Autodesk Inventor part; units mm, degrees
ref_plane "Work Plane4" through (0, 0, -5) normal (0, 0, 1) x (1, 0, 0)
ref_plane "YZ Plane" through (0, 0, 0) normal (1, 0, 0) x (0, 1, 0)
ref_plane "XZ Plane" through (0, 0, 0) normal (0, 1, 0) x (-1, 0, 0)
sketch "Sketch1" plane through (0, 0, 0) normal (0, 0, 1) x (1, 0, 0)
  circle A0 centre (0, 0) radius 71.5
  circle A1 centre (0, 0) radius 73.5
  circle A2 centre (0, 0) radius 81.5
  circle A3 centre (0, 0) radius 83.5
  circle A4 centre (0, 0) radius 91.5
  circle A5 centre (0, 0) radius 93.5
  circle A6 centre (0, 0) radius 52.5
  circle A7 centre (0, 0) radius 62.5
  dimension "d0" = 143
  dimension "d1" = 147
  dimension "d2" = 163
  dimension "d3" = 167
  dimension "d4" = 183
  dimension "d5" = 187
  dimension "d6" = 105
  dimension "d7" = 125
extrude "Extrusion1" add sketch "Sketch1" along normal blind 10
extrude "Extrusion2" add sketch "Sketch1" against normal blind 10 contours A0 | A1 | A2 | A3 | A4 | A5 | A6 | A7
extrude "Extrusion3" cut sketch "Sketch1" against normal blind 10 contours A6
ref_plane "Work Plane4" through (0, 0, -5) normal (0, 0, 1) x (1, 0, 0)
ref_plane "Work Plane3" through (0, 0, 0) normal (0, 0, 1) x (1, 0, 0)
sketch "Sketch3" plane through (0, 0, 10) normal (0, 0, 1) x (1, 0, 0)
  circle A0 centre (0, 0) radius 61
  dimension "d18" = 122
sketch "Sketch4" plane through (0, 0, 5) normal (0, 0, 1) x (1, 0, 0)
  circle A0 centre (0, 0) radius 61
  dimension "d19" = 122
sketch "Sketch5" plane through (0, 0, 0) normal (0, 0, 1) x (1, 0, 0)
  circle A0 centre (0, 0) radius 61
  dimension "d20" = 122
ref_plane "Work Plane1" through (0, 0, 10) normal (0, 0, 1) x (1, 0, 0)
ref_plane "Work Plane2" through (0, 0, 5) normal (0, 0, 1) x (1, 0, 0)
properties part number "labyrinth"
Geometry: final body of the model. Coordinates: model frame, mm. A direction names the side the tool comes from. Coordinates: 2 decimals unless noted, no trailing zeros. Loops run counter-clockwise (first coordinate to the right, second up) from the corner with the lowest first, then second, coordinate; pieces in that order, holes last. Notation, with made-up numbers: (47, 60.25) -> (83, 60.25) arc R19 cw to (83, 72.25) -> close; hole circle Ø9 at (52.25, 0.25). An arc over 180 degrees is marked (long way). Use a Markdown table: item, result. Add a question column.
(1) Line query: line 1 along Y through (x, z) = (1.5, -2); line 2 along X through (y, z) = (-2, -5.5); line 3 along Z through (x, y) = (-9, -68.5). Output: solid intervals per line, ascending.
(2) Pin query (flat end, axial travel): pin 1 Ø3 at (y, z) = (58, 1.5) entering from +X; pin 2 Ø10 at (x, y) = (44.5, -22.5) entering from +Z; pin 3 Ø1 at (x, z) = (42.5, 1.5) entering from +Y; pin 4 Ø3 at (x, z) = (2.5, -3.5) entering from -Y. Return the tip coordinate at first contact, or that it passes through.
(3) Section query D-D, the plane y = -60. Return loops of the section in (x, z), plus the area to 3 significant figures.
(4) Access query for faces 4 (the cylindrical face through (-52.7, -48.32, 4.93)), 5 (the flat face through (69, -62, 10)). Directions: +Z, -Z, +X, -X, +Y, -Y. A direction counts if a zero-diameter tool reaches every point of the face in a straight line with its end or side. Return the directions, or none.
(5) Mould query, pull axis X, two halves, no side actions, for faces 1 (the flat face through (40, -40, -10)), 2 (the cylindrical face through (50.265, -78.84, -0.14)), 3 (the cylindrical face through (-15.933, 71.752, 4.93)). Classes: pulls with the +X half, pulls with the -X half, needs draft (parallel to the pull), parting line crosses it, or undercut.
(6) Section query C-C, the plane z = -4. Return loops of the section in (x, y).
Answer:
| question | item | result |
|---|---|---|
| 1 | line 1 | y = -93.49 to -52.48, 52.48 to 93.49 |
| 1 | line 2 | x = -93.48 to -52.46, 52.46 to 93.48 |
| 1 | line 3 | z = -10 to 0 |
| 2 | pin 1 | stops at x = 74.5 |
| 2 | pin 2 | stops at z = 10 |
| 2 | pin 3 | stops at y = 83.54 |
| 2 | pin 4 | stops at y = -93.49 |
| 3 | outline | (-71.71, -10) -> (71.71, -10) -> (71.71, 10) -> (69.08, 10) -> (69.08, 0) -> (58.07, 0) -> (58.07, 10) -> (55.16, 10) -> (55.16, 0) -> (42.45, 0) -> (42.45, 10) -> (38.89, 10) -> (38.89, 0) -> (17.5, 0) -> (17.5, 10) -> (-17.5, 10) -> (-17.5, 0) -> (-38.89, 0) -> (-38.89, 10) -> (-42.45, 10) -> (-42.45, 0) -> (-55.16, 0) -> (-55.16, 10) -> (-58.07, 10) -> (-58.07, 0) -> (-69.08, 0) -> (-69.08, 10) -> (-71.71, 10) -> close |
| 3 | area | 1,970 mm^2 |
| 4 | face 4 | +Z |
| 4 | face 5 | +Z, +X, -X, +Y, -Y |
| 5 | face 1 | needs draft |
| 5 | face 2 | parting line crosses it |
| 5 | face 3 | undercut |
| 6 | outline | circle Ø187 at (0, 0); hole circle Ø105 at (0, 0) |
